For this review, take the finished solid that the model builds, in its own axes (mm). A direction names the side the tool comes from. Round coordinates to 2 decimals unless told otherwise and drop trailing zeros. Order: outer loops, then holes, each group sorted by start corner. A loop starts at its lowest first (then second) coordinate and runs counter-clockwise, first axis right, second up.
```python
from build123d import *

# Parameters (mm, degrees)
SKETCH2_W                = 40
SKETCH2_H                = 70
BOSS_EXTRUDE1_DEPTH      = 43.5
SKETCH4_R                = 16.5
BOSS_EXTRUDE2_DEPTH      = 25
M3_CLEARANCE_HOLE1_D     = 3.2
M3_CLEARANCE_HOLE1_DEPTH = 3.18
M3_CLEARANCE_HOLE1_TIP   = 0.96137699


with BuildPart() as part:
    # Sketch2 → Boss-Extrude1 (new body)
    with BuildSketch(Plane(origin=(0, 0, 0), x_dir=(1, 0, 0), z_dir=(0, 1, 0))):
        Rectangle(SKETCH2_W, SKETCH2_H)
    extrude(amount=BOSS_EXTRUDE1_DEPTH)

    # Sketch4 → Boss-Extrude2 (add)
    with BuildSketch(Plane.XY.offset(35)):
        with Locations((0, 23)):
            Circle(SKETCH4_R)
    extrude(amount=BOSS_EXTRUDE2_DEPTH)

    # M3 Clearance Hole1
    with Locations(Plane(origin=(0, 0, 0), x_dir=(-1, 0, 0), z_dir=(0, -1, 0))):
        with Locations((-7, 20), (7, 20), (7, -25), (-7, -25)):
            Hole(M3_CLEARANCE_HOLE1_D / 2, depth=M3_CLEARANCE_HOLE1_DEPTH)
            with Locations((0, 0, -(M3_CLEARANCE_HOLE1_DEPTH + M3_CLEARANCE_HOLE1_TIP / 2))):  # 118° drill point
                Cone(0, M3_CLEARANCE_HOLE1_D / 2, M3_CLEARANCE_HOLE1_TIP, mode=Mode.SUBTRACT)


solid = part.part
```
Q1. Take a section at B-B, the plane z = 36. State the section outline as (x, y) points.
Q2. Take a section at C-C, the plane y = 15.5. State the section outline as (x, z) points.
Q3. Clearance check with flat-ended pins moving along their axes: pin 1 (4 mm diameter, centred on y = 29, z = 46.5, fed in from +X); pin 2 (1.9 mm diameter, centred on x = 7, z = -20, fed in from -Y); pin 3 (2 mm diameter, centred on x = -1.5, z = 48.5, fed in from -Y). State where each tip first meets the part, or that it passes through.
Q4. Take a section at A-A, the plane x = 0. State the section outline as (y, z) points.
Q5. Wall thickness on line 1 (Z direction, x = 7, y = 1); line 2 (X direction, y = 1, z = -20); line 3 (Z direction, x = 10.5, y = 3.5): over which ranges is each line inside the solid? List them lowest first.
Q6. Mouldability with a two-part tool opening along Z and no side actions: class faces 3 (the face through (-5, 7, 35)), 4 (the face through (-3.577, 6.892, 47.325)), 5 (the face through (6.792, 1.612, 23.414)) as +Z half, -Z half, draft (parallel to the pull), parting line (faces both ways), or undercut.
Q7. Tool access review of faces 1 (the face through (-7.208, 1.612, -21.586)), 2 (the face through (20, 21, 0)): name each direction out of +Z, -Z, +X, -X, +Y, -Y from which nothing blocks a thin tool from reaching the whole face with its end or side.
Working result:
1. outline: circle Ø33 at (0, 23)
2. outline: (-20, -35) - (20, -35) - (20, 35) - (14.7, 35) - (14.7, 60) - (-14.7, 60) - (-14.7, 35) - (-20, 35) - close
3. pin 1: stops at x = 16.01
3. pin 2: stops at y = 3.57
3. pin 3: stops at y = 6.51
4. outline: (0, -35) - (43.5, -35) - (43.5, 35) - (39.5, 35) - (39.5, 60) - (6.5, 60) - (6.5, 35) - (0, 35) - close
5. line 1: z = -35 to -21.6, -18.4 to 23.4, 26.6 to 35
5. line 2: x = -20 to -8.6, -5.4 to 5.4, 8.6 to 20
5. line 3: z = -35 to 35
6. face 3: +Z half
6. face 4: draft
6. face 5: undercut
7. face 1: -Y
7. face 2: +Z, -Z, +X, +Y, -Y
